from build123d import *

# Parameters (mm, degrees)
F0_R     = 12.7
F1_DEPTH = 12.7
F3_D     = 22.86
F4_R     = 15.875
F5_DEPTH = 1.905
F7_D     = 22.86


with BuildPart() as f1:
    # F0 (on Top) → F1 (new body)
    with BuildSketch(Plane.XY):
        Circle(F0_R)
    extrude(amount=F1_DEPTH)

    # F3 (through all)
    with Locations(Plane.XY.offset(14.605)):
        with Locations((0, 0)):
            Hole(F3_D / 2)

    # F4 (on face) → F5 (join)
    with BuildSketch(Plane.XY.offset(12.7)):
        Circle(F4_R)
    extrude(amount=F5_DEPTH)

    # F7 (through all)
    with Locations(Plane.XY.offset(12.7)):
        with Locations((0, 0)):
            Hole(F7_D / 2)


solid = f1.part
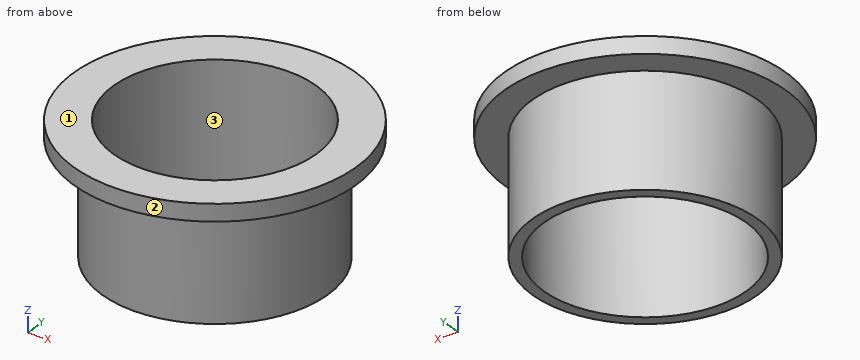
Geometry: final body of the model. Coordinates: model frame, mm. Face numbers are marked on the shaded views. Round coordinates to 2 decimals unless told otherwise and drop trailing zeros. Loops run counter-clockwise (first coordinate to the right, second up) from the corner with the lowest first, then second, coordinate; pieces in that order, holes last. Notation, with made-up numbers: (-24, 48) - (7, 48) arc R20 cw to (7, 71) - close; hole circle Ø2 at (48, 69). An arc over 180 degrees is marked (long way). Write each question's results on one line, items separated by ' | '. Start each with the question number.
1) Cut plane C-C on z = 8.5. Return loops of the section in (x, y).
2) Line query: probe 1 along Y at (x, z) = (0, 8); probe 2 along Y at (x, z) = (0, 12.75) (3 decimals); probe 3 along Z at (x, y) = (9, 13) (3 decimals). Output: solid intervals per line, ascending. Write a range as [from, to].
3) Cut plane A-A on x = 0. Return loops of the section in (y, z) (3 decimals).
4) Cut plane D-D on x = 12. Return loops of the section in (y, z) (3 decimals).
5) Mould query, pull axis X, two halves, no side actions, for the marked faces 1, 2 and 3. Classes: released by +X, released by -X, zero draft, split by the parting line, or undercut.
6) First-contact query: P1, Ø1.5, axis at y = -0.5, z = 10.5, coming from the +X side; P2, Ø1, axis at x = -11.5, z = 2.5, coming from the +Y side; P3, Ø6, axis at x = -2, y = 10, coming from the -Z side; P4, Ø8, axis at x = -4.5, z = 2, coming from the +Y side. Flat tips, straight axial feed; report the tip coordinate or a pass-through.
Verdict:
1) outline: circle Ø25.4 at (0, 0); hole circle Ø22.86 at (0, 0)
2) probe 1: y = [-12.7, -11.43], [11.43, 12.7] | probe 2: y = [-15.875, -11.43], [11.43, 15.875] | probe 3: z = [12.7, 14.605]
3) outline: (-15.875, 12.7) - (-12.7, 12.7) - (-12.7, 0) - (-11.43, 0) - (-11.43, 14.605) - (-15.875, 14.605) - close; (11.43, 0) - (12.7, 0) - (12.7, 12.7) - (15.875, 12.7) - (15.875, 14.605) - (11.43, 14.605) - close
4) outline: (-10.393, 12.7) - (-4.158, 12.7) - (-4.158, 0) - (4.158, 0) - (4.158, 12.7) - (10.393, 12.7) - (10.393, 14.605) - (-10.393, 14.605) - close
5) face 1: zero draft | face 2: split by the parting line | face 3: undercut
6) P1: stops at x = 12.7 | P2: stops at y = 6.35 | P3: stops at z = 0 | P4: stops at y = 12.69
